Geometry: final body of the model. Coordinates: model frame, mm. A direction names the side the tool comes from. Give positions to 0.01 mm unless a question says otherwise; leave off trailing zeros. Loops run counter-clockwise (first coordinate to the right, second up) from the corner with the lowest first, then second, coordinate; pieces in that order, holes last. Notation, with made-up numbers: M 56,10.25 L 80,10.25 A36 cw 80,46.25 Z; hole C 65.5,23.5 d6. An arc over 180 degrees is marked long. Put each result on its own line as item: value.
```python
from build123d import *

# Parameters (mm, degrees)
SKETCH2_R               = 75
SKETCH2_R_2             = 67.5
BOSS_EXTRUDE2_DEPTH     = 10
BOSS_EXTRUDE3_DEPTH     = 80
BOSS_EXTRUDE4_DEPTH     = 15
BOSS_EXTRUDE5_DEPTH     = 10
SKETCH7_W               = 10
SKETCH7_H               = 10
BOSS_EXTRUDE6_DEPTH     = 137
SKETCH8_R               = 62.5
CUT_EXTRUDE1_DEPTH      = 150
SKETCH9_R               = 1.5
CUT_EXTRUDE2_DEPTH      = 6.5
SKETCH10_R              = 1.5
CUT_EXTRUDE3_DEPTH      = 152.5
CUT_EXTRUDE3_DEPTH_BACK = 6.5
SKETCH12_R              = 1.5
CUT_EXTRUDE4_DEPTH      = 6.5
CUT_EXTRUDE4_DEPTH_BACK = 6.5
SKETCH13_R              = 1.5
CUT_EXTRUDE5_DEPTH      = 6.5
CUT_EXTRUDE5_DEPTH_BACK = 6.5
SKETCH14_R              = 1.5
CUT_EXTRUDE6_DEPTH      = 6.5
CUT_EXTRUDE6_DEPTH_BACK = 6.5
CUT_EXTRUDE7_DEPTH      = 4


with BuildPart() as part:
    # Sketch2 → Boss-Extrude2 (new body)
    with BuildSketch(Plane.XY):
        Circle(SKETCH2_R)
        Circle(SKETCH2_R_2, mode=Mode.SUBTRACT)
    extrude(amount=BOSS_EXTRUDE2_DEPTH)

    # Sketch3 → Boss-Extrude3 (add)
    with BuildSketch(Plane.XY.offset(10)):
        with BuildLine():
            Line((75, 0), (67.5, 0))
            ThreePointArc((67.5, 0), (0, -67.5), (-67.5, 0))
            Line((-67.5, 0), (-75, 0))
            ThreePointArc((-75, 0), (0, -75), (75, 0))
        make_face()
    extrude(amount=BOSS_EXTRUDE3_DEPTH)

    # Sketch5 → Boss-Extrude4 (add)
    with BuildSketch(Plane.XY.offset(10)):
        with BuildLine():
            ThreePointArc((-47.877777695, -40.174225605), (-54.126587737, -31.25), (-58.730788799, -21.376258958))
            Line((-58.730788799, -21.376258958), (-63.429251903, -23.086359674))
            ThreePointArc((-63.429251903, -23.086359674), (-58.456714755, -33.75), (-51.707999911, -43.388163654))
            Line((-51.707999911, -43.388163654), (-47.877777695, -40.174225605))
        make_face()
        with BuildLine():
            ThreePointArc((10.853011104, -61.550484563), (0, -62.5), (-10.853011104, -61.550484563))
            Line((-10.853011104, -61.550484563), (-11.721251993, -66.474523328))
            ThreePointArc((-11.721251993, -66.474523328), (0, -67.5), (11.721251993, -66.474523328))
            Line((11.721251993, -66.474523328), (10.853011104, -61.550484563))
        make_face()
        with BuildLine():
            Line((63.429251903, -23.086359674), (58.730788799, -21.376258958))
            ThreePointArc((58.730788799, -21.376258958), (54.126587737, -31.25), (47.877777695, -40.174225605))
            Line((47.877777695, -40.174225605), (51.707999911, -43.388163654))
            ThreePointArc((51.707999911, -43.388163654), (58.456714755, -33.75), (63.429251903, -23.086359674))
        make_face()
    extrude(amount=BOSS_EXTRUDE4_DEPTH)

    # Sketch6 → Boss-Extrude5 (add)
    with BuildSketch(Plane.XY.offset(65)):
        with BuildLine():
            ThreePointArc((-47.877777695, -40.174225605), (-54.126587737, -31.25), (-58.730788799, -21.376258958))
            Line((-58.730788799, -21.376258958), (-63.429251903, -23.086359674))
            ThreePointArc((-63.429251903, -23.086359674), (-58.456714755, -33.75), (-51.707999911, -43.388163654))
            Line((-51.707999911, -43.388163654), (-47.877777695, -40.174225605))
        make_face()
        with BuildLine():
            ThreePointArc((10.853011104, -61.550484563), (0, -62.5), (-10.853011104, -61.550484563))
            Line((-10.853011104, -61.550484563), (-11.721251993, -66.474523328))
            ThreePointArc((-11.721251993, -66.474523328), (0, -67.5), (11.721251993, -66.474523328))
            Line((11.721251993, -66.474523328), (10.853011104, -61.550484563))
        make_face()
        with BuildLine():
            Line((63.429251903, -23.086359674), (58.730788799, -21.376258958))
            ThreePointArc((58.730788799, -21.376258958), (54.126587737, -31.25), (47.877777695, -40.174225605))
            Line((47.877777695, -40.174225605), (51.707999911, -43.388163654))
            ThreePointArc((51.707999911, -43.388163654), (58.456714755, -33.75), (63.429251903, -23.086359674))
        make_face()
    extrude(amount=BOSS_EXTRUDE5_DEPTH)

    # Sketch7 → Boss-Extrude6 (add)
    with BuildSketch(Plane.ZY.offset(-67.5)):
        with Locations((70, -5)):
            Rectangle(SKETCH7_W, SKETCH7_H)
    extrude(amount=BOSS_EXTRUDE6_DEPTH)

    # Sketch8 → Cut-Extrude1 (cut)
    with BuildSketch(Plane.XY.offset(10)):
        Circle(SKETCH8_R)
    extrude(amount=CUT_EXTRUDE1_DEPTH, mode=Mode.SUBTRACT)

    # Sketch9 → Cut-Extrude2 (cut)
    with BuildSketch(Plane(origin=(0, 0, 0), x_dir=(1, 0, 0), z_dir=(0, 1, 0))):
        with Locations((-68.75, -70)):
            Circle(SKETCH9_R)
        with Locations((68.75, -70)):
            Circle(SKETCH9_R)
    extrude(amount=-CUT_EXTRUDE2_DEPTH, mode=Mode.SUBTRACT)

    # Sketch10 → Cut-Extrude3 (cut, two sides)
    with BuildSketch(Plane.ZY.offset(-67.5)) as cut_extrude3_sk:
        with Locations((84, -6)):
            Circle(SKETCH10_R)
    extrude(amount=CUT_EXTRUDE3_DEPTH, mode=Mode.SUBTRACT)
    extrude(cut_extrude3_sk.sketch, amount=-CUT_EXTRUDE3_DEPTH_BACK, mode=Mode.SUBTRACT)

    # Sketch12 → Cut-Extrude4 (cut, two sides)
    with BuildSketch(Plane(origin=(0, -67.5, 0), x_dir=(1, 0, 0), z_dir=(0, 1, 0))) as cut_extrude4_sk:
        with Locations((0, -84)):
            Circle(SKETCH12_R)
    extrude(amount=CUT_EXTRUDE4_DEPTH, mode=Mode.SUBTRACT)
    extrude(cut_extrude4_sk.sketch, amount=-CUT_EXTRUDE4_DEPTH_BACK, mode=Mode.SUBTRACT)

    # Sketch13 → Cut-Extrude5 (cut, two sides)
    with BuildSketch(Plane(origin=(-33.75, -58.456714755, 0), x_dir=(0.866025404, -0.5, 0), z_dir=(0.5, 0.866025404, 0))) as cut_extrude5_sk:
        with Locations((0.543285245, -70)):
            Circle(SKETCH13_R)
    extrude(amount=CUT_EXTRUDE5_DEPTH, mode=Mode.SUBTRACT)
    extrude(cut_extrude5_sk.sketch, amount=-CUT_EXTRUDE5_DEPTH_BACK, mode=Mode.SUBTRACT)

    # Sketch14 → Cut-Extrude6 (cut, two sides)
    with BuildSketch(Plane(origin=(33.75, -58.456714755, 0), x_dir=(0.866025404, 0.5, 0), z_dir=(-0.5, 0.866025404, 0))) as cut_extrude6_sk:
        with Locations((-0.543285245, -70)):
            Circle(SKETCH14_R)
    extrude(amount=CUT_EXTRUDE6_DEPTH, mode=Mode.SUBTRACT)
    extrude(cut_extrude6_sk.sketch, amount=-CUT_EXTRUDE6_DEPTH_BACK, mode=Mode.SUBTRACT)

    # Sketch15 → Cut-Extrude7 (cut)
    with BuildSketch(Plane.XY.offset(10)):
        with BuildLine():
            ThreePointArc((71.25, 0), (0, 71.25), (-71.25, 0))
            Line((-71.25, 0), (-67.5, 0))
            ThreePointArc((-67.5, 0), (0, 67.5), (67.5, 0))
            Line((67.5, 0), (71.25, 0))
        make_face()
    extrude(amount=-CUT_EXTRUDE7_DEPTH, mode=Mode.SUBTRACT)


solid = part.part
```
Item 1: Section A-A on z = 14.5. Output: boundary loops of the cut face in (x, y).
Output values:
outline: M -75,0 A75 ccw 75,0 L 67.5,0 A67.5 cw 63.43,-23.09 L 58.73,-21.38 A62.5 cw 47.88,-40.17 L 51.71,-43.39 A67.5 cw 11.72,-66.47 L 10.85,-61.55 A62.5 cw -10.85,-61.55 L -11.72,-66.47 A67.5 cw -51.71,-43.39 L -47.88,-40.17 A62.5 cw -58.73,-21.38 L -63.43,-23.09 A67.5 cw -67.5,0 Z
Item 2: Section B-B on y = 17. Output: boundary loops of the cut face in (x, z), then the cut area to 3 significant figures.
Output values:
outline: M -73.05,0 L -65.32,0 L -65.32,6 L -69.19,6 L -69.19,10 L -73.05,10 Z; M 65.32,0 L 73.05,0 L 73.05,10 L 69.19,10 L 69.19,6 L 65.32,6 Z
area: 124 mm²
Item 3: Section C-C on x = -18.5. Output: boundary loops of the cut face in (y, z).
Output values:
outline: M -72.68,0 L -64.92,0 L -64.92,90 L -72.68,90 Z; M 64.92,0 L 72.68,0 L 72.68,10 L 68.81,10 L 68.81,6 L 64.92,6 Z
Item 4: Pin query (flat end, axial travel): pin 1 Ø3.5 at (y, z) = (-6, 84) entering from -X; pin 2 Ø8 at (x, y) = (53.5, -34) entering from -Z; pin 3 Ø4 at (y, z) = (-33.5, 47) entering from +X; pin 4 Ø17 at (x, y) = (-57, -32) entering from -Z. Return the tip coordinate at first contact, or that it passes through.
Output values:
pin 1: x = -74.88
pin 2: z = 10
pin 3: x = 68.06
pin 4: z = 0
Item 5: Section D-D on y = 48. Output: boundary loops of the cut face in (x, z).
Output values:
outline: M -57.63,0 L -47.46,0 L -47.46,6 L -52.66,6 L -52.66,10 L -57.63,10 Z; M 47.46,0 L 57.63,0 L 57.63,10 L 52.66,10 L 52.66,6 L 47.46,6 Z
Item 6: Set-up query: faces 5 (the flat face through (56, -33, 10)), 6 (the flat face through (-65, -5, 65)), 7 (the flat face through (-61.05, -22.22, 17.4)), 8 (the flat face through (-56, -32, 65)), 9 (the flat face through (-64, -10, 70)). Return all of +Z, -Z, +X, -X, +Y, -Y with unobstructed straight access to the full face (end or side cutting, diameter ignored); none if empty.
Output values:
face 5: -Z
face 6: -Z, +Y
face 7: +Z, -Z, +Y
face 8: +Y
face 9: +Z, -Z
Item 7: Mould query, pull axis Z, two halves, no side actions, for faces 1 (the flat face through (-11.28, -63.98, 69.93)), 2 (the flat face through (65, -5, 75)), 3 (the flat face through (-56, -32, 25)), 4 (the flat face through (56, -33, 65)). Classes: pulls with the +Z half, pulls with the -Z half, needs draft (parallel to the pull), parting line crosses it, or undercut.
Output values:
face 1: needs draft
face 2: pulls with the +Z half
face 3: undercut
face 4: undercut
Item 8: Line query: probe 1 along X at (y, z) = (-2.5, 70); probe 2 along Z at (x, y) = (0, -72.5); probe 3 along Z at (x, y) = (-54.5, 46.5). Output: solid intervals per line, ascending. Write a range as [from, to].
Output values:
probe 1: [-74.96, -70.25], [-67.25, -62.45], [62.45, 67.25], [70.25, 74.96]
probe 2: [0, 82.5], [85.5, 90]
probe 3: [0, 10]
